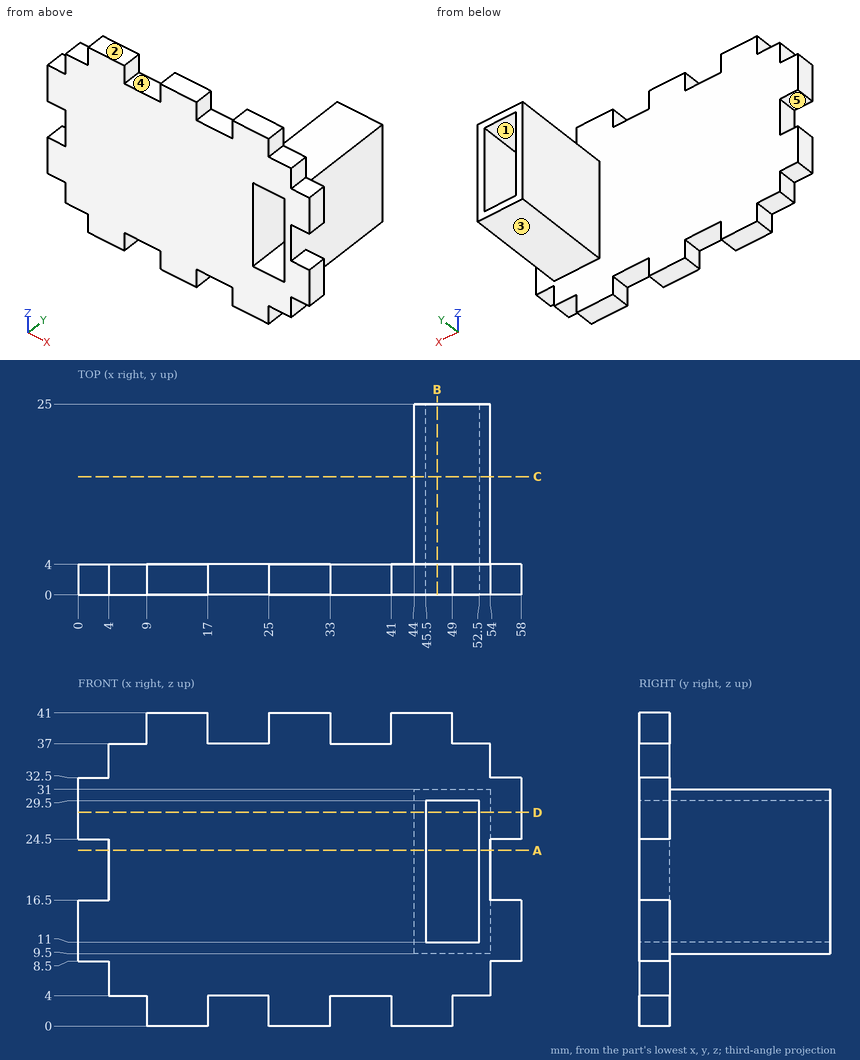
Check sheet for the drawn part. Datum: minimum x, y, z corner. Units: mm. A direction names the side the tool comes from. Round coordinates to 2 decimals unless told otherwise and drop trailing zeros. Order: outer loops, then holes, each group sorted by start corner. A loop starts at its lowest first (then second) coordinate and runs counter-clockwise, first axis right, second up. Notation, with made-up numbers: (28.25, 30.25) -> (71.25, 30.25) arc R26 ccw to (71.25, 69.25) -> close; hole circle Ø9 at (-24, 20). An arc over 180 degrees is marked (long way). Put each result on its own line as item: value. Start each with the question number.
(1) Section check D-D (z = 28). Enter the section's corners in (x, y).
(2) Section check A-A (z = 23). Enter the section's corners in (x, y), then the cut area to 3 significant figures.
(3) Section check B-B (x = 47). Enter the section's corners in (y, z), then the cut area to 3 significant figures.
(4) Draft check along X on the marked faces 1 and 2. Enter one of: +X half, -X half, draft (parallel to the pull), parting line (faces both ways), or undercut.
(5) Material ranges on line 1 along X through (y, z) = (2.75, 20.5); line 2 along X through (y, z) = (14, 11.5); line 3 along Y through (x, z) = (44, 8), recorded low to high.
(6) Section check C-C (y = 15.5). Enter the section's corners in (x, z), then the cut area to 3 significant figures.
(7) Tool access check on the marked faces 3, 4 and 5. Record the directions out of +Z, -Z, +X, -X, +Y, -Y that give a thin tool (end or side, any length) a straight path to the whole face; none if there is none.
(8) Depth check by flat-ended pin: pin 1 Ø1.2 at (y, z) = (3, 7) entering from +X; pin 2 Ø12 at (x, z) = (38.5, 34) entering from -Y; pin 3 Ø4.5 at (x, y) = (55.5, 1) entering from -Z; pin 4 Ø2 at (y, z) = (1, 38.5) entering from +X. Enter the tip coordinate at first touch or a pass-through.
Completed:
1. outline: (0, 0) -> (45.5, 0) -> (45.5, 25) -> (44, 25) -> (44, 4) -> (0, 4) -> close; (52.5, 0) -> (58, 0) -> (58, 4) -> (54, 4) -> (54, 25) -> (52.5, 25) -> close
2. outline: (4, 0) -> (45.5, 0) -> (45.5, 25) -> (44, 25) -> (44, 4) -> (4, 4) -> close; (52.5, 0) -> (54, 0) -> (54, 25) -> (52.5, 25) -> close
2. area: 235 mm2
3. outline: (0, 0) -> (4, 0) -> (4, 9.5) -> (25, 9.5) -> (25, 11) -> (0, 11) -> close; (0, 29.5) -> (25, 29.5) -> (25, 31) -> (4, 31) -> (4, 41) -> (0, 41) -> close
3. area: 153 mm2
4. face 1: undercut
4. face 2: draft
5. line 1: x = 4 to 45.5, 52.5 to 54
5. line 2: x = 44 to 45.5, 52.5 to 54
5. line 3: y = 0 to 4
6. outline: (44, 9.5) -> (54, 9.5) -> (54, 31) -> (44, 31) -> close; hole (45.5, 11) -> (52.5, 11) -> (52.5, 29.5) -> (45.5, 29.5) -> close
6. area: 85.5 mm2
7. face 3: -Z, +X, -X, +Y
7. face 4: +Z, +Y, -Y
7. face 5: -X, +Y, -Y
8. pin 1: stops at x = 54
8. pin 2: stops at y = 0
8. pin 3: stops at z = 4
8. pin 4: stops at x = 49
